Here's how the part is built. I have some questions about the finished solid (model axes, mm). Give positions to 0.01 mm unless a question says otherwise; leave off trailing zeros. Write each loop counter-clockwise with the first axis right and the second up, starting at its lowest first coordinate (ties: lowest second). Pieces come first, ordered by that corner, then holes. Notation, with made-up numbers: (35.5, 76) -> (54.5, 76) arc R25 cw to (54.5, 99) -> close; hole circle Ø9 at (-28.5, 24.5). An arc over 180 degrees is marked (long way). Use CSV: the item, a comma, the result in double quotes. Start each with the question number.
(1) If we mould it in two halves opening along Y, with no side actions, what happens to faces 1 (the flat face through (0, 0, 0.6)), 2 (the cylindrical face through (3.195, -5.623, 0.296)), 3 (the cylindrical face through (-1.658, -7.468, 0.296))? For each: pulls with the +Y half, pulls with the -Y half, needs draft (parallel to the pull), parting line crosses it, or undercut.
(2) Suppose I cut it at D-D on y = -3.5. List the corners of the cut face in (x, z) for me.
(3) I need wall thicknesses on L1, parallel to Y at x = -6.25, z = 0.35; L2, parallel to Y at x = 1, z = 0.3; L3, parallel to X at y = 2.75, z = 0.2. Which ranges of each line are inside material? Lowest first, please. Write a range as [from, to].
(4) Suppose I cut it at A-A on z = 0.5. List the corners of the cut face in (x, y) for me.
(5) Suppose I cut it at C-C on y = -6.4. List the corners of the cut face in (x, z) for me.
(6) Suppose I cut it at B-B on x = 6. List the corners of the cut face in (y, z) for me, plus the area to 3 significant figures.
from build123d import *

# Parameters (mm, degrees)
SKETCH1_R           = 7.65
BOSS_EXTRUDE1_DEPTH = 0.6


with BuildPart() as part:
    # Sketch1 → Boss-Extrude1 (new body)
    with BuildSketch(Plane.XY):
        Circle(SKETCH1_R)
        with BuildLine():
            ThreePointArc((0, 5.6), (0.8, 6.4), (0, 7.2))
            ThreePointArc((0, 7.2), (-1.404650319, 7.061654019), (-2.755320713, 6.651932634))
            ThreePointArc((-2.755320713, 6.651932634), (-3.188277593, 5.606682262), (-2.143027221, 5.173725382))
            ThreePointArc((-2.143027221, 5.173725382), (-1.092505803, 5.49239757), (0, 5.6))
        make_face(mode=Mode.SUBTRACT)
        with BuildLine():
            ThreePointArc((6.651932634, 2.755320713), (5.606682262, 3.188277593), (5.173725382, 2.143027221))
            ThreePointArc((5.173725382, 2.143027221), (5.49239757, 1.092505803), (5.6, 0))
            ThreePointArc((5.6, 0), (6.4, -0.8), (7.2, 0))
            ThreePointArc((7.2, 0), (7.061654019, 1.404650319), (6.651932634, 2.755320713))
        make_face(mode=Mode.SUBTRACT)
        with BuildLine():
            ThreePointArc((2.755320713, -6.651932634), (3.188277593, -5.606682262), (2.143027221, -5.173725382))
            ThreePointArc((2.143027221, -5.173725382), (1.092505803, -5.49239757), (0, -5.6))
            ThreePointArc((0, -5.6), (-0.8, -6.4), (0, -7.2))
            ThreePointArc((0, -7.2), (1.404650319, -7.061654019), (2.755320713, -6.651932634))
        make_face(mode=Mode.SUBTRACT)
        with BuildLine():
            ThreePointArc((-6.651932634, -2.755320713), (-5.606682262, -3.188277593), (-5.173725382, -2.143027221))
            ThreePointArc((-5.173725382, -2.143027221), (-5.49239757, -1.092505803), (-5.6, 0))
            ThreePointArc((-5.6, 0), (-6.4, 0.8), (-7.2, 0))
            ThreePointArc((-7.2, 0), (-7.061654019, -1.404650319), (-6.651932634, -2.755320713))
        make_face(mode=Mode.SUBTRACT)
    extrude(amount=BOSS_EXTRUDE1_DEPTH)


solid = part.part
Geometry says:
1,face 1,"needs draft"
1,face 2,"undercut"
1,face 3,"parting line crosses it"
2,outline,"(-6.8, 0) -> (6.8, 0) -> (6.8, 0.6) -> (-6.8, 0.6) -> close"
3,L1,"[-4.41, -3.17], [0.79, 4.41]"
3,L2,"[-7.58, -7.13], [-5.51, 7.58]"
3,L3,"[-7.14, 5.17], [6.65, 7.14]"
4,outline,"circle Ø15.3 at (0, 0); hole (-7.2, 0) arc R7.2 ccw to (-6.65, -2.76) arc R0.8 ccw to (-5.17, -2.14) arc R5.6 cw to (-5.6, 0) arc R0.8 ccw to start; hole (-2.76, 6.65) arc R0.8 ccw to (-2.14, 5.17) arc R5.6 cw to (0, 5.6) arc R0.8 ccw to (0, 7.2) arc R7.2 ccw to start; hole (0, -7.2) arc R7.2 ccw to (2.76, -6.65) arc R0.8 ccw to (2.14, -5.17) arc R5.6 cw to (0, -5.6) arc R0.8 ccw to start; hole (5.17, 2.14) arc R5.6 cw to (5.6, 0) arc R0.8 ccw to (7.2, 0) arc R7.2 ccw to (6.65, 2.76) arc R0.8 ccw to start"
5,outline,"(-4.19, 0) -> (-0.8, 0) -> (-0.8, 0.6) -> (-4.19, 0.6) -> close; (3.08, 0) -> (4.19, 0) -> (4.19, 0.6) -> (3.08, 0.6) -> close"
6,outline,"(-4.75, 0) -> (-0.69, 0) -> (-0.69, 0.6) -> (-4.75, 0.6) -> close; (3.24, 0) -> (4.75, 0) -> (4.75, 0.6) -> (3.24, 0.6) -> close"
6,area,"3.33 mm²"
